from build123d import *

# Parameters (mm, degrees)
F0_W     = 600
F0_H     = 600
F1_DEPTH = 900
F2_W     = 600
F2_H     = 100
F3_DEPTH = 40
F4_W     = 600
F4_H     = 800
F5_DEPTH = 35
F7_DEPTH = 300


with BuildPart() as f1:
    # F0 (on Top) → F1 (new body)
    with BuildSketch(Plane.XY):
        Rectangle(F0_W, F0_H)
    extrude(amount=F1_DEPTH)

    # F2 (on face) → F3 (cut)
    with BuildSketch(Plane.XZ.offset(300)):
        with Locations((0, 50)):
            Rectangle(F2_W, F2_H)
    extrude(amount=-F3_DEPTH, mode=Mode.SUBTRACT)

    # F4 (on face) → F5 (cut)
    with BuildSketch(Plane.XZ.offset(300)):
        with Locations((0, 500)):
            Rectangle(F4_W, F4_H)
    extrude(amount=-F5_DEPTH, mode=Mode.SUBTRACT)

    # F6 (on Right) → F7 (join, symmetric)
    with BuildSketch(Plane.YZ):
        Polygon((-296.1448182649, 92.6515106829), (-265, 100), (-255.2672442922, 102.2964029116), (-257.5636472038, 112.0291586194), (-267.2964029116, 109.7327557078), (-448.7122329282, 878.6204566235), (-479.8570511932, 871.2719673063), align=None)
    extrude(amount=F7_DEPTH, both=True)


solid = f1.part
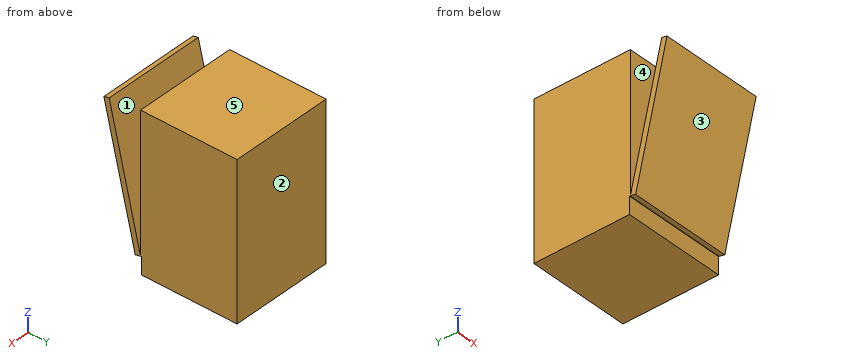
Input: part model. Units: mm. Frame: model coordinates. Face numbers are marked on the shaded views. A direction names the side the tool comes from. Coordinates: 2 decimals unless noted, no trailing zeros. Order: outer loops, then holes, each group sorted by start corner. A loop starts at its lowest first (then second) coordinate and runs counter-clockwise, first axis right, second up. Notation, with made-up numbers: M 17.25,20.25 L 74.25,20.25 A23 ccw 74.25,56.25 Z; hole C 26,-29 d3. An arc over 180 degrees is marked long. Write item = value, one per line. Start each with the question number.
(1) Section A-A on x = -76.5. Output: boundary loops of the cut face in (y, z).
(2) Section C-C on z = 76. Output: boundary loops of the cut face in (x, y).
(3) Line query: line 1 along Y through (x, z) = (-227, 267.5); line 2 along Y through (x, z) = (73.5, 771.5); line 3 along Y through (x, z) = (-94, 100.5). Output: solid intervals per line, ascending. Write a range as [from, to].
(4) Section D-D on y = -423.5. Output: boundary loops of the cut face in (x, z).
(5) Pull-direction query (Y, two-part tool) for the marked faces 1, 2 and 3; classes: released by +Y, released by -Y, zero draft, split by the parting line, or undercut.
(6) Section B-B on z = 228. Output: boundary loops of the cut face in (x, y).
(7) First-contact query: P1, Ø2.5, axis at x = -133, y = -261.5, coming from the -Z side; P2, Ø3, axis at x = -3.5, z = 202.5, coming from the -Y side. Flat tips, straight axial feed; report the tip coordinate or a pass-through.
(8) Reachability of the marked faces 4 and 5 from +Z, -Z, +X, -X, +Y, -Y: full face, straight path, thin tool, end or side. Return the list, or none.
Result set:
q1.outline = M -479.86,871.27 L -296.14,92.65 L -265,100 L -260,100 L -260,0 L 300,0 L 300,900 L -265,900 L -265,110.27 L -267.3,109.73 L -448.71,878.62 Z
q2.outline = M -300,-260 L 300,-260 L 300,300 L -300,300 Z
q3.line_1 = [-337.4, -304.52], [-265, 300]
q3.line_2 = [-456.32, -423.44], [-265, 300]
q3.line_3 = [-298, 300]
q4.outline = M -300,632.42 L 300,632.42 L 300,771.76 L -300,771.76 Z
q5.face_1 = undercut
q5.face_2 = released by +Y
q5.face_3 = released by -Y
q6.outline = M -300,-328.08 L 300,-328.08 L 300,-295.2 L -300,-295.2 Z; M -300,-265 L 300,-265 L 300,300 L -300,300 Z
q7.P1 = 100
q7.P2 = -322.42
q8.face_4 = +Z, +X, -X
q8.face_5 = +Z, +X, -X, +Y, -Y
